Autodesk Inventor part; units mm, degrees
ref_plane "YZ Plane" through (0, 0, 0) normal (1, 0, 0) x (0, 1, 0)
ref_plane "XZ Plane" through (0, 0, 0) normal (0, 1, 0) x (-1, 0, 0)
ref_plane "XY Plane" through (0, 0, 0) normal (0, 0, 1) x (1, 0, 0)
sketch "Sketch2" plane through (0, 0, 0) normal (0, 0, 1) x (1, 0, 0)
  line L0 (0, -11.2) -> (0, 11.2)
  line L1 (-3.6, 8) -> (-3.6, -8)
  line L2 (-3.6, -8) -> (-3.2, -8)
  line L3 (-3.2, -8) -> (-3.2, -7.2)
  line L4 (-3.2, -7.2) -> (-2.4, -7.2)
  line L5 (-2.4, -7.2) -> (-2.4, -0.8)
  line L6 (-2.4, -0.8) -> (-3.2, -0.8)
  line L7 (-3.2, -0.8) -> (-3.2, 0.8)
  line L8 (-3.2, 0.8) -> (-2.4, 0.8)
  line L9 (-2.4, 0.8) -> (-2.4, 7.2)
  line L10 (-2.4, 7.2) -> (-3.2, 7.2)
  line L11 (-3.2, 7.2) -> (-3.2, 8)
  line L12 (-3.2, 8) -> (-3.6, 8)
  point P0 (0, 0)
  point P1 (-3.2, 0)
  dimension "d0" = 16
  dimension "d1" = 6.4
  dimension "d2" = 7.2
  dimension "d3" = 4.8
  dimension "d4" = 0.8
  dimension "d5" = 1.6
revolve "Revolution1" add sketch "Sketch2" angle 360 about axis through (0, -10, 0) along (0, 1, 0)
sketch "Sketch3" plane through (0, 0, 0) normal (0, 1, 0) x (-1, 0, 0)
  circle A0 centre (0, 0) radius 3.2
  circle A1 centre (0, 0) radius 3.6
  line L0 (-3.2, 0) -> (-3.2, 1.6492)
  line L1 (3.2, 0) -> (3.2, 1.6492)
extrude "Extrusion1" cut sketch "Sketch3" along normal up to surface (1.6 mm away) from surface at -0.8 contours A0 L0 A1 L1 picked at (-0.1286, 3.4412)
equation "\"d0\" = 2 * lu"
equation "\"d1\" = tsd"
equation "\"d2\" = tlad"
equation "\"d3\" = tpd"
equation "\"d4\" = tsl"
equation "\"d5\" = 2 * tsl"
properties part number "62462-LtBluishGray" material "ABS Plastic"
Geometry check sheet. Reference: the model listing, model coordinates, mm. A direction names the side the tool comes from. Give positions to 0.01 mm unless a question says otherwise; leave off trailing zeros. Loops run counter-clockwise (first coordinate to the right, second up) from the corner with the lowest first, then second, coordinate; pieces in that order, holes last. Notation, with made-up numbers: M 33,-38.5 L 88,-38.5 A13 ccw 88,-33.5 Z; hole C 2.5,-11 d1. An arc over 180 degrees is marked long. Write item = value, one per line. Start each with the question number.
1. Section check A-A, the plane x = 0. Enter the section's corners in (y, z), plus the area to 3 significant figures.
2. Section check B-B, the plane z = 0.25. Enter the section's corners in (x, y), plus the area to 3 significant figures.
3. Tool access check on faces 1 (the face through (0, 0.8, 3)), 2 (the face through (2.539, -7.594, -1.947)), 3 (the face through (-1.29, 4.045, 2.024)). Record the directions out of +Z, -Z, +X, -X, +Y, -Y that give a thin tool (end or side, any length) a straight path to the whole face; none if there is none.
4. Section check C-C, the plane y = 2.5. Enter the section's corners in (x, z).
5. Section check D-D, the plane x = 3. Enter the section's corners in (y, z), plus the area to 3 significant figures.
6. Draft check along Z on faces 4 (the face through (2.539, 7.606, -1.947)), 5 (the face through (-3.2, 0, 1)), 6 (the face through (0.1, 0, -3.2)). Enter one of: +Z half, -Z half, draft (parallel to the pull), parting line (faces both ways), or undercut.
7. Thickness scan on probe 1 along Y at (x, z) = (-3, 1); probe 2 along Z at (x, y) = (0, 7.4); probe 3 along Z at (x, y) = (0, -2.75). Record the ranges inside material, lowest first.
8. Go/stop test with flat-tipped pins: P1, Ø0.5, axis at y = 0.5, z = 1, coming from the +X side; P2, Ø4, axis at x = 3, y = -0.5, coming from the +Z side; P3, Ø1, axis at x = -1.5, y = -5, coming from the -Z side; P4, Ø4, axis at x = 1, z = -2.5, coming from the +Y side. Record where each tip stops, or that it passes through.
Values follow:
q1.outline = M -8,-3.6 L 8,-3.6 L 8,-3.2 L 7.2,-3.2 L 7.2,-2.4 L 0.8,-2.4 L 0.8,-3.2 L -0.8,-3.2 L -0.8,-2.4 L -7.2,-2.4 L -7.2,-3.2 L -8,-3.2 Z; M -8,3.2 L -7.2,3.2 L -7.2,2.4 L -0.8,2.4 L -0.8,3.6 L -8,3.6 Z; M 0.8,2.4 L 7.2,2.4 L 7.2,3.2 L 8,3.2 L 8,3.6 L 0.8,3.6 Z
q1.area = 32.6 mm^2
q2.outline = M -3.59,-8 L -3.19,-8 L -3.19,-7.2 L -2.39,-7.2 L -2.39,-0.8 L -3.2,-0.8 L -3.2,0.8 L -2.39,0.8 L -2.39,7.2 L -3.19,7.2 L -3.19,8 L -3.59,8 Z; M 2.39,-7.2 L 3.19,-7.2 L 3.19,-8 L 3.59,-8 L 3.59,8 L 3.19,8 L 3.19,7.2 L 2.39,7.2 L 2.39,0.8 L 3.2,0.8 L 3.2,-0.8 L 2.39,-0.8 Z
q2.area = 33.4 mm^2
q3.face_1 = +Z
q3.face_2 = -Y
q3.face_3 = +Y, -Y
q4.outline = C 0,0 d7.2; hole C 0,0 d4.8
q5.outline = M -8,-1.99 L 8,-1.99 L 8,-1.11 L 7.2,-1.11 L 7.2,1.11 L 8,1.11 L 8,1.99 L 0.8,1.99 L 0.8,-1.11 L -0.8,-1.11 L -0.8,1.99 L -8,1.99 L -8,1.11 L -7.2,1.11 L -7.2,-1.11 L -8,-1.11 Z
q5.area = 55.2 mm^2
q6.face_4 = undercut
q6.face_5 = draft
q6.face_6 = +Z half
q7.probe_1 = -7.2 to -0.8, 0.8 to 7.2
q7.probe_2 = -3.6 to -3.2, 3.2 to 3.6
q7.probe_3 = -3.6 to -2.4, 2.4 to 3.6
q8.P1 = 3.52
q8.P2 = 3.45
q8.P3 = -3.46
q8.P4 = 8
